Design review of the part built by this model. Coordinates are the model's own, in mm. Give positions to 0.01 mm unless a question says otherwise; leave off trailing zeros. Order: outer loops, then holes, each group sorted by start corner. A loop starts at its lowest first (then second) coordinate and runs counter-clockwise, first axis right, second up. Notation, with made-up numbers: M 48.5,36 L 94.5,36 A19 cw 94.5,73 Z; hole C -18.75,12.5 d8. An arc over 180 degrees is marked long. Answer as a JSON object with one key per item and string values.
from build123d import *

# Parameters (mm, degrees)
ESQUISSE1_R                  = 160
ESQUISSE1_R_2                = 50
BOSS_EXTRU_1_DEPTH           = 5
ESQUISSE2_R                  = 7.5
ENL_V_MAT_EXTRU_1_DEPTH      = 11
ESQUISSE3_W                  = 16.5
ESQUISSE3_H                  = 25
ENL_V_MAT_EXTRU_2_DEPTH      = 11
ESQUISSE4_R                  = 6.5
ENL_V_MAT_EXTRU_3_DEPTH      = 11
R_P_TITION_CIRCULAIRE1_COUNT = 5
R_P_TITION_CIRCULAIRE2_COUNT = 20


with BuildPart() as part:
    # Esquisse1 → Boss.-Extru.1 (new body, symmetric)
    with BuildSketch(Plane.XY):
        Circle(ESQUISSE1_R)
        Circle(ESQUISSE1_R_2, mode=Mode.SUBTRACT)
    extrude(amount=BOSS_EXTRU_1_DEPTH, both=True)

    # Esquisse2 → Enlèv. mat.-Extru.1 (cut, through all)
    with BuildSketch(Plane.XY.offset(5)):
        with Locations((-10.011805763, 63.212053798)):
            Circle(ESQUISSE2_R)
    enl_v_mat_extru_1 = extrude(amount=-ENL_V_MAT_EXTRU_1_DEPTH, mode=Mode.SUBTRACT)

    # Esquisse3 → Enlèv. mat.-Extru.2 (cut, through all)
    with BuildSketch(Plane.XY.offset(5)):
        with Locations((0, 147.5)):
            Rectangle(ESQUISSE3_W, ESQUISSE3_H)
    enl_v_mat_extru_2 = extrude(amount=-ENL_V_MAT_EXTRU_2_DEPTH, mode=Mode.SUBTRACT)

    # Esquisse4 → Enlèv. mat.-Extru.3 (cut, through all)
    with BuildSketch(Plane.XY.offset(5)):
        with Locations((-20.80578385, 131.362549299)):
            Circle(ESQUISSE4_R)
    enl_v_mat_extru_3 = extrude(amount=-ENL_V_MAT_EXTRU_3_DEPTH, mode=Mode.SUBTRACT)

    # Répétition circulaire1: Enlèv. mat.-Extru.1, Enlèv. mat.-Extru.3 ×5 about axis
    r_p_tition_circulaire1_axis = Axis((0, 0, 0), (0, 0, 1))
    add([enl_v_mat_extru_1.rotate(r_p_tition_circulaire1_axis, i * 360 / R_P_TITION_CIRCULAIRE1_COUNT) for i in range(1, R_P_TITION_CIRCULAIRE1_COUNT)], mode=Mode.SUBTRACT)
    add([enl_v_mat_extru_3.rotate(r_p_tition_circulaire1_axis, i * 360 / R_P_TITION_CIRCULAIRE1_COUNT) for i in range(1, R_P_TITION_CIRCULAIRE1_COUNT)], mode=Mode.SUBTRACT)

    # Répétition circulaire2: Enlèv. mat.-Extru.2 ×20 about axis
    r_p_tition_circulaire2_axis = Axis((0, 0, 0), (0, 0, 1))
    for i in range(1, R_P_TITION_CIRCULAIRE2_COUNT):
        add(enl_v_mat_extru_2.rotate(r_p_tition_circulaire2_axis, i * 360 / R_P_TITION_CIRCULAIRE2_COUNT), mode=Mode.SUBTRACT)


solid = part.part
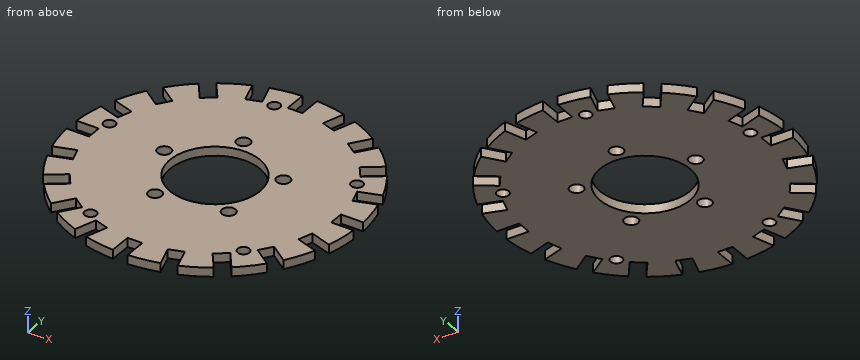
(1) We need section C-C (x = 140). Write out the cut boundary in (y, z).
Checked values:
{"outline": "M -77.46,-5 L -54.16,-5 L -54.16,5 L -77.46,5 Z; M -36.81,-5 L -8.25,-5 L -8.25,5 L -36.81,5 Z; M 8.25,-5 L 36.81,-5 L 36.81,5 L 8.25,5 Z; M 54.16,-5 L 77.46,-5 L 77.46,5 L 54.16,5 Z"}
(2) We need section D-D (z = -1.75). Count the separate pieces of the cut face and the enclosed holes in it, plus the area to 3 significant figures.
Checked values:
{"separate pieces": "1", "enclosed holes": "11", "area": "62,800 mm^2"}
(3) To check wall thickness, follow L1, parallel to X at y = -140.5, z = -3; L2, parallel to Y at x = -122, z = -1.75; L3, parallel to Y at x = 84, z = 3.5. State the ranges of each line that lie inside material, in increasing order. Write a range as from..to.
Checked values:
{"L1": "x = -76.55..-54.33, -36.98..-8.25, 8.25..36.98, 54.33..76.55", "L2": "y = -103.52..-98.84, -78.44..78.44, 98.84..103.52", "L3": "y = -136.18..-129.65, -105.84..105.84, 129.65..136.18"}
(4) We need section B-B (y = 119). Write out the cut boundary in (x, z).
Checked values:
{"outline": "M -106.95,-5 L -96.66,-5 L -96.66,5 L -106.95,5 Z; M -76.26,-5 L 76.26,-5 L 76.26,5 L -76.26,5 Z; M 96.66,-5 L 106.95,-5 L 106.95,5 L 96.66,5 Z"}
(5) Insertion check: pin 1 (1.5 mm diameter, centred on y = -102, z = 4, fed in from -X); pin 2 (3 mm diameter, centred on y = 2, z = -2.5, fed in from -X); pin 3 (3 mm diameter, centred on x = 0.5, z = -0.5, fed in from -Y). Each pin has a flat end and moves straight along its axis. Give the tip position at first contact, or say it passes through.
Checked values:
{"pin 1": "stops at x = -123.89", "pin 2": "stops at x = -135", "pin 3": "stops at y = -135"}
(6) We need section A-A (x = 30). Write out the cut boundary in (y, z), plus the area to 3 significant figures.
Checked values:
{"outline": "M -157.16,-5 L -40,-5 L -40,5 L -157.16,5 Z; M 40,-5 L 157.16,-5 L 157.16,5 L 40,5 Z", "area": "2,340 mm^2"}
